Autodesk Inventor part; units mm, degrees
ref_plane "YZ Plane" through (0, 0, 0) normal (1, 0, 0) x (0, 1, 0)
ref_plane "XZ Plane" through (0, 0, 0) normal (0, 1, 0) x (-1, 0, 0)
ref_plane "XY Plane" through (0, 0, 0) normal (0, 0, 1) x (1, 0, 0)
sketch "Szkic1" plane through (0, 0, 0) normal (0, 1, 0) x (-1, 0, 0)
  circle A0 centre (0, 0) radius 22.5
  dimension "d0" = 45
extrude "Wyciągnięcie proste1" add sketch "Szkic1" along normal blind 21
sketch "Szkic2" plane through (0, 21, 0) normal (0, 1, 0) x (1, 0, 0)
  circle A0 centre (0, 0) radius 22.5
  line L0 (22.1151, -4.144) -> (29.5, -3.5)
  line L1 (29.5, -3.5) -> (29.5, 3.5)
  line L2 (29.5, 3.5) -> (22.1151, 4.144)
  line L3 (22.1151, -4.144) -> (22.1151, 4.144)
  dimension "d3" = 7
  dimension "d4" = 7
extrude "Wyciągnięcie proste2" add sketch "Szkic2" against normal blind 21 contours A0 L2 L1 L0
fillet "Zaokrąglenie1" radius 3 2 edges at (29.5, 10.5, -3.5) (29.5, 10.5, 3.5)
pattern_circular "Szyk kołowy2" count 9 over 360 about axis through (0, 0, 0) along (0, 1, 0) of "Wyciągnięcie proste2", "Zaokrąglenie1"
sketch "Szkic3" plane through (0, 0, 0) normal (0, -1, 0) x (1, 0, 0)
  point P0 (0, 0)
sketch "Szkic4" plane through (0, 21, 0) normal (0, 1, 0) x (1, 0, 0)
  circle A0 centre (0, 0) radius 1.5
  line L0 (-1.118, 1) -> (1.118, 1)
  circle A1 centre (0, 0) radius 2
  dimension "d14" = 3
  dimension "d15" = 2.5
  dimension "d16" = 0
  dimension "d17" = 0
extrude "Wyciągnięcie proste3" cut sketch "Szkic4" against normal through all contours A0 L0 picked at (0.0594, 0.1702)
properties part number "KOŁO"
The listing builds one solid part. Answer for the finished solid, in the listing's coordinates (mm). A direction names the side the tool comes from. Coordinates: 2 decimals unless noted, no trailing zeros. Write each loop counter-clockwise with the first axis right and the second up, starting at its lowest first coordinate (ties: lowest second). Pieces come first, ordered by that corner, then holes. Notation, with made-up numbers: (51.25, 24.25) - (82.25, 24.25) arc R25 ccw to (82.25, 41.25) - close; hole circle Ø11 at (-33, 32). An arc over 180 degrees is marked (long way). Return JSON: item names as keys, results as strings. Group by question number.
Q1. The part is cut by section C-C on z = -8. Write down the section's boundary in (x, y).
Q2. The part is cut by section A-A on z = 0. Write down the section's boundary in (x, y).
Q3. Find the intervals of material crossed by line 1 along Z through (x, y) = (-16, 6.5); line 2 along X through (y, z) = (8.5, 0); line 3 along X through (y, z) = (6.75, 17.5), in increasing order. Write a range as [from, to].
Q4. Flat-ended cylindrical pins translate along their axes: pin 1 Ø1.8 at (x, z) = (0, 0) entering from +Y; pin 2 Ø2 at (y, z) = (4, 11) entering from +X; pin 3 Ø4 at (x, y) = (-7, 18) entering from +Z; pin 4 Ø10 at (x, y) = (-11.5, 16.5) entering from +Z. Find the tip coordinate at first contact, or state that the pin passes through.
Q5. The part is cut by section B-B on x = 20.5. Write down the section's boundary in (y, z), and give its area (3 significant figures).
Q6. Which of the six approach directions +Z, -Z, +X, -X, +Y, -Y give full straight-line access (tool end or side, diameter ignored) to faces 4 (the flat face through (0.37, 10.65, -24.78)), 5 (the flat face through (21.231, 10.647, -12.666)), 6 (the flat face through (0, 11, -1)), 7 (the flat face through (1, 0, -6))?
Q7. For a pull along X with two mould halves and no side action, classify faces 1 (the cylindrical face through (21.16, 10.35, 7.65)), 2 (the cylindrical face through (-22.5, 10.4, 0.1)), 3 (the cylindrical face through (20.24, 10.35, 20.58)) as +X half, -X half, draft (parallel to the pull), parting line (faces both ways), or undercut.
Evaluation:
{
 "1": {"outline": "(-28.14, 0) - (21.03, 0) - (21.03, 21) - (-28.14, 21) - close"},
 "2": {"outline": "(-22.5, 0) - (-1.5, 0) - (-1.5, 21) - (-22.5, 21) - close; (1.5, 0) - (29.5, 0) - (29.5, 21) - (1.5, 21) - close"},
 "3": {"line 1": "z = [-24.72, -19.98], [-15.82, 15.82], [19.98, 24.72]", "line 2": "x = [-22.5, -1.5], [1.5, 29.5]", "line 3": "x = [-14.84, 14.14], [14.43, 23.6]"},
 "4": {"pin 1": "passes through", "pin 2": "stops at x = 20.56", "pin 3": "stops at z = 23.41", "pin 4": "stops at z = 26.32"},
 "5": {"outline": "(0, -20.53) - (21, -20.53) - (21, -11.94) - (0, -11.94) - close; (0, -9.27) - (21, -9.27) - (21, 9.27) - (0, 9.27) - close; (0, 11.94) - (21, 11.94) - (21, 20.53) - (0, 20.53) - close", "area": "750 mm2"},
 "6": {"face 4": "-Z, +Y, -Y", "face 5": "+X, +Y, -Y", "face 6": "+Y, -Y", "face 7": "+Z, -Z, +X, -X, -Y"},
 "7": {"face 1": "+X half", "face 2": "-X half", "face 3": "undercut"}
}
